Could you check a few things on this model? Use its own coordinates, in mm. Give positions to 0.01 mm unless a question says otherwise; leave off trailing zeros. Order: outer loops, then holes, each group sorted by start corner. A loop starts at its lowest first (then second) coordinate and runs counter-clockwise, first axis right, second up. Notation, with made-up numbers: (-29, -14.75) - (-3, -14.75) arc R12 cw to (-3, 0.25) - close; hole circle Ø1 at (31.25, -30.75). An arc over 180 degrees is marked (long way). One line per question, with ' | ' between items. Start each with the question number.
1. Imagine slicing it at A-A (z = 0). Please give me the cut outline in (x, y).
2. Imagine slicing it at C-C (z = -6.5). Please give me the cut outline in (x, y), and give its area (3 significant figures).
3. I need wall thicknesses on probe 1 along Y at (x, z) = (1.45, 0); probe 2 along Z at (x, y) = (4.65, 5.25); probe 3 along Z at (x, y) = (0.35, -4.25). Which ranges of each line are inside material? Lowest first, please. Write a range as from..to.
4. Imagine slicing it at B-B (y = -7). Please give me the cut outline in (x, z), and give its area (3 significant figures).
5. Imagine slicing it at D-D (z = 6.25). Please give me the cut outline in (x, y).
6. For P1, Ø3, axis at x = 4.5, y = 5.5, coming from the +Z side, with a flat end and sliding along its axis, tell me the tip position at first contact or that it passes through.
7. If we mould it in two halves opening along Z, with no side actions, what happens to faces 1 (the flat face through (6, -4, 0)), 2 (the cylindrical face through (2.96, 4.54, -3.32)), 3 (the cylindrical face through (2.958, -7.385, 1.262))? For each: released by +Z, released by -Z, zero draft, split by the parting line, or undercut.
```python
from build123d import *

# Parameters (mm, degrees)
BASPROSKE_W        = 12
BASPROSKE_H        = 9
TOOTHCUT_DEPTH     = 18.492855685
TEETHCUTS_COUNT    = 10
TEETHCUTS_ANGLE    = 324
BORSKE_R           = 0.4
BORE_DEPTH         = 50.0000508
SKETCH1_R          = 3
SKETCH1_R_2        = 0.4
CUT_EXTRUDE2_DEPTH = 18.298122882
SKETCH2_R          = 20.440784698
CUT_EXTRUDE3_DEPTH = 6


with BuildPart() as part:
    # BasProSke → Base-Revolve (revolve)
    with BuildSketch(Plane(origin=(0, 0, 0), x_dir=(1, 0, 0), z_dir=(0, 1, 0)), mode=Mode.PRIVATE) as base_revolve_sk:
        with Locations((6, 4.5)):
            Rectangle(BASPROSKE_W, BASPROSKE_H)
    revolve(base_revolve_sk.sketch.rotate(Axis((-10, 0, 0), (1, 0, 0)), 180), axis=Axis((-10, 0, 0), (1, 0, 0)))

    # TooCutSke → ToothCut (cut, through all)
    with BuildSketch(Plane(origin=(0, 0, 0), x_dir=(0, 0, -1), z_dir=(1, 0, 0))):
        with BuildLine():
            ThreePointArc((0.883878355, 5.554109745), (0, 5.624), (-0.883878355, 5.554109745))
            ThreePointArc((-0.883878355, 5.554109745), (-1.258245767, 7.379188248), (-2.637816971, 8.631324741))
            ThreePointArc((-2.637816971, 8.631324741), (0, 9.0254), (2.637816971, 8.631324741))
            ThreePointArc((2.637816971, 8.631324741), (1.258245767, 7.379188248), (0.883878355, 5.554109745))
        make_face()
    toothcut = extrude(amount=TOOTHCUT_DEPTH, mode=Mode.SUBTRACT)

    # TeethCuts: ToothCut ×10 about axis
    teethcuts_axis = Axis((-10, 0, 0), (1, 0, 0))
    for i in range(1, TEETHCUTS_COUNT):
        add(toothcut.rotate(teethcuts_axis, i * TEETHCUTS_ANGLE / (TEETHCUTS_COUNT - 1)), mode=Mode.SUBTRACT)

    # BorSke → Bore (cut, symmetric)
    with BuildSketch(Plane(origin=(0, 0, 0), x_dir=(0, 0, -1), z_dir=(1, 0, 0))):
        with Locations(Location((0, 0, 0), (0, 0, 180))):
            Circle(BORSKE_R)
    extrude(amount=BORE_DEPTH, both=True, mode=Mode.SUBTRACT)

    # Sketch1 → Cut-Extrude2 (cut, through all)
    with BuildSketch(Plane.ZY):
        Circle(SKETCH1_R)
        Circle(SKETCH1_R_2, mode=Mode.SUBTRACT)
    extrude(amount=-CUT_EXTRUDE2_DEPTH, mode=Mode.SUBTRACT)

    # Sketch2 → Cut-Extrude3 (cut)
    with BuildSketch(Plane(origin=(12, 0, 0), x_dir=(0, 0, -1), z_dir=(1, 0, 0))):
        Circle(SKETCH2_R)
    extrude(amount=-CUT_EXTRUDE3_DEPTH, mode=Mode.SUBTRACT)


solid = part.part
```
Results found:
1) outline: (0, -5.62) - (6, -5.62) - (6, -3) - (0, -3) - close; (0, 3) - (6, 3) - (6, 5.62) - (0, 5.62) - close
2) outline: (0, -5.5) - (6, -5.5) - (6, -3.34) - (0, -3.34) - close; (0, -1.13) - (6, -1.13) - (6, 1.13) - (0, 1.13) - close; (0, 3.34) - (6, 3.34) - (6, 5.5) - (0, 5.5) - close | area: 39.4 mm2
3) probe 1: y = -5.62..-3, 3..5.62 | probe 2: z = -7.31..-5.4, -2.75..2.75, 5.4..7.31 | probe 3: z = -7.14..-4.16, -3.68..3.68, 4.16..7.14
4) outline: (0, -3.34) - (6, -3.34) - (6, -1.08) - (0, -1.08) - close; (0, 1.08) - (6, 1.08) - (6, 3.34) - (0, 3.34) - close | area: 27.1 mm2
5) outline: (0, -5.48) - (6, -5.48) - (6, -3.13) - (0, -3.13) - close; (0, -1.1) - (6, -1.1) - (6, 1.1) - (0, 1.1) - close; (0, 3.13) - (6, 3.13) - (6, 5.48) - (0, 5.48) - close
6) P1: stops at z = 7.39
7) face 1: zero draft | face 2: undercut | face 3: undercut
